from build123d import *

# Parameters (mm, degrees)
SKETCH1_W           = 100
SKETCH1_H           = 38.1
SKETCH1_R           = 2.54
BOSS_EXTRUDE1_DEPTH = 6.35
SKETCH2_W           = 100
SKETCH2_H           = 38.1
BOSS_EXTRUDE2_DEPTH = 2.54


with BuildPart() as part:
    # Sketch1 → Boss-Extrude1 (new body)
    with BuildSketch(Plane(origin=(0, 0, 0), x_dir=(1, 0, 0), z_dir=(0, 1, 0))):
        with Locations((28.74, 0)):
            Rectangle(SKETCH1_W, SKETCH1_H)
        Circle(SKETCH1_R, mode=Mode.SUBTRACT)
        with Locations((57.48, 0)):
            Circle(SKETCH1_R, mode=Mode.SUBTRACT)
    extrude(amount=BOSS_EXTRUDE1_DEPTH)

    # Sketch2 → Boss-Extrude2 (add)
    with BuildSketch(Plane(origin=(0, 6.35, 0), x_dir=(1, 0, 0), z_dir=(0, 1, 0))):
        with Locations((28.74, 0)):
            Rectangle(SKETCH2_W, SKETCH2_H)
    extrude(amount=-BOSS_EXTRUDE2_DEPTH)


solid = part.part
Part model, mm, in its own coordinate system. A direction names the side the tool comes from. Coordinates: 2 decimals unless noted, no trailing zeros. Loops run counter-clockwise (first coordinate to the right, second up) from the corner with the lowest first, then second, coordinate; pieces in that order, holes last. Notation, with made-up numbers: (-27, 20.25) - (10, 20.25) arc R32 cw to (10, 58.25) - close; hole circle Ø9 at (39.25, -24). An arc over 180 degrees is marked (long way). Write each question's results on one line, items separated by ' | '. Start each with the question number.
Q1. Slice it at A-A on z = 0. Give the cut face in (x, y), and give its area (3 significant figures).
Q2. Probe line 1 along X through (y, z) = (1.1, 0); line 2 along Z through (x, y) = (0, 2.1); line 3 along X through (y, z) = (2, 1.5). List the from-to ranges inside material, lowest first.
Q3. Two-plate mould, pull along Z, no slides. Class faces 1 (the flat face through (28, 3, 19.05)), 2 (the cylindrical face through (-0.33, 1.88, -2.52)), 3 (the flat face through (28, 3, -19.05)): +Z half, -Z half, draft (parallel to the pull), parting line (faces both ways), or undercut.
Q4. Which spindle directions (+Z, -Z, +X, -X, +Y, -Y) get a long thin tool onto all of the face, cutting with end or side? Do faces 4 (the cylindrical face through (54.942, 1.878, -0.112)), 5 (the flat face through (78.74, 3, 0)). Say none if no direction does.
Q5. Slice it at B-B on x = 0. Give the cut face in (y, z).
Answer:
1) outline: (-21.26, 0) - (-2.54, 0) - (-2.54, 3.81) - (2.54, 3.81) - (2.54, 0) - (54.94, 0) - (54.94, 3.81) - (60.02, 3.81) - (60.02, 0) - (78.74, 0) - (78.74, 6.35) - (-21.26, 6.35) - close | area: 596 mm2
2) line 1: x = -21.26 to -2.54, 2.54 to 54.94, 60.02 to 78.74 | line 2: z = -19.05 to -2.54, 2.54 to 19.05 | line 3: x = -21.26 to -2.05, 2.05 to 55.43, 59.53 to 78.74
3) face 1: +Z half | face 2: undercut | face 3: -Z half
4) face 4: -Y | face 5: +Z, -Z, +X, +Y, -Y
5) outline: (0, -19.05) - (6.35, -19.05) - (6.35, 19.05) - (0, 19.05) - (0, 2.54) - (3.81, 2.54) - (3.81, -2.54) - (0, -2.54) - close
